from build123d import *

# Parameters (mm, degrees)
SALIENTE_EXTRUIR1_DEPTH = 111
SALIENTE_EXTRUIR2_DEPTH = 5
CROQUIS3_W              = 20
CROQUIS3_H              = 5
SALIENTE_EXTRUIR3_DEPTH = 2
SALIENTE_EXTRUIR4_DEPTH = 5
SALIENTE_EXTRUIR5_DEPTH = 2
CROQUIS6_R              = 2
CORTAR_EXTRUIR1_DEPTH   = 41
CROQUIS7_R              = 4
CORTAR_EXTRUIR2_DEPTH   = 4
CORTAR_EXTRUIR4_DEPTH   = 118


with BuildPart() as part:
    # Croquis1 → Saliente-Extruir1 (new body)
    with BuildSketch(Plane.XY):
        with BuildLine():
            Line((0, 5), (0, 0))
            Line((0, 0), (28, 0))
            ThreePointArc((28, 0), (29.414213562, 0.585786438), (30, 2))
            Line((30, 2), (30, 13))
            ThreePointArc((30, 13), (29.414213562, 14.414213562), (28, 15))
            Line((28, 15), (0, 15))
            Line((0, 15), (0, 10))
            Line((0, 10), (20, 10))
            Line((20, 10), (20, 5))
            Line((20, 5), (0, 5))
        make_face()
    extrude(amount=SALIENTE_EXTRUIR1_DEPTH)

    # Croquis2 → Saliente-Extruir2 (add)
    with BuildSketch(Plane.XY.offset(111)):
        with BuildLine():
            Line((20, 15), (20, 10))
            Line((20, 10), (20, 5))
            Line((20, 5), (0, 5))
            Line((0, 5), (0, 0))
            Line((0, 0), (28, 0))
            ThreePointArc((28, 0), (29.414213562, 0.585786438), (30, 2))
            Line((30, 2), (30, 13))
            ThreePointArc((30, 13), (29.414213562, 14.414213562), (28, 15))
            Line((28, 15), (20, 15))
        make_face()
    extrude(amount=SALIENTE_EXTRUIR2_DEPTH)

    # Croquis3 → Saliente-Extruir3 (add)
    with BuildSketch(Plane.XY.offset(116)):
        Polygon((20, 10), (20, 15), (11, 15), (0, 15), (0, 10), align=None)
        with BuildLine():
            Line((28, 15), (20, 15))
            Line((20, 15), (20, 10))
            Line((20, 10), (20, 5))
            Line((20, 5), (0, 5))
            Line((0, 5), (0, 0))
            Line((0, 0), (28, 0))
            ThreePointArc((28, 0), (29.414213562, 0.585786438), (30, 2))
            Line((30, 2), (30, 13))
            ThreePointArc((30, 13), (29.414213562, 14.414213562), (28, 15))
        make_face()
        with Locations((10, 7.5)):
            Rectangle(CROQUIS3_W, CROQUIS3_H)
    extrude(amount=SALIENTE_EXTRUIR3_DEPTH)

    # Croquis4 → Saliente-Extruir4 (add)
    with BuildSketch(Plane(origin=(0, 0, 0), x_dir=(-1, 0, 0), z_dir=(0, 0, -1))):
        with BuildLine():
            Line((-20, 5), (-20, 10))
            Line((-20, 10), (-20, 15))
            Line((-20, 15), (-28, 15))
            ThreePointArc((-28, 15), (-29.414213562, 14.414213562), (-30, 13))
            Line((-30, 13), (-30, 2))
            ThreePointArc((-30, 2), (-29.414213562, 0.585786438), (-28, 0))
            Line((-28, 0), (0, 0))
            Line((0, 0), (0, 5))
            Line((0, 5), (-20, 5))
        make_face()
    extrude(amount=SALIENTE_EXTRUIR4_DEPTH)

    # Croquis5 → Saliente-Extruir5 (add)
    with BuildSketch(Plane(origin=(0, 0, -5), x_dir=(-1, 0, 0), z_dir=(0, 0, -1))):
        with BuildLine():
            Line((0, 15), (-28, 15))
            ThreePointArc((-28, 15), (-29.414213562, 14.414213562), (-30, 13))
            Line((-30, 13), (-30, 2))
            ThreePointArc((-30, 2), (-29.414213562, 0.585786438), (-28, 0))
            Line((-28, 0), (0, 0))
            Line((0, 0), (0, 15))
        make_face()
    extrude(amount=SALIENTE_EXTRUIR5_DEPTH)

    # Croquis6 → Cortar-Extruir1 (cut)
    with BuildSketch(Plane.XZ):
        with Locations((5, 24.25)):
            Circle(CROQUIS6_R)
        with Locations((5, 86.75)):
            Circle(CROQUIS6_R)
    extrude(amount=-CORTAR_EXTRUIR1_DEPTH, mode=Mode.SUBTRACT)

    # Croquis7 → Cortar-Extruir2 (cut)
    with BuildSketch(Plane(origin=(0, 0, 0), x_dir=(-1, 0, 0), z_dir=(0, -1, 0))):
        with Locations((-5, -24.25)):
            Circle(CROQUIS7_R)
        with Locations((-5, -86.75)):
            Circle(CROQUIS7_R)
    extrude(amount=-CORTAR_EXTRUIR2_DEPTH, mode=Mode.SUBTRACT)

    # Croquis9 → Cortar-Extruir4 (cut)
    with BuildSketch(Plane.XY.offset(118)):
        Polygon((27.046454018, 15), (28.719274454, 12.085683765), (24.239354869, 9.549004814), (21.152820727, 15), align=None)
    extrude(amount=-CORTAR_EXTRUIR4_DEPTH, mode=Mode.SUBTRACT)


solid = part.part
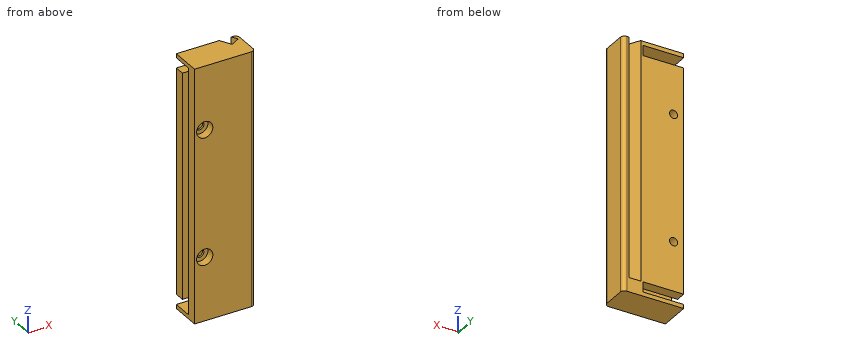
Build history of the part. All positions in model axes, mm. Give positions to 0.01 mm unless a question says otherwise; leave off trailing zeros. Loops run counter-clockwise (first coordinate to the right, second up) from the corner with the lowest first, then second, coordinate; pieces in that order, holes last. Notation, with made-up numbers: (-24.5, -32) -> (-14.5, -32) arc R18 ccw to (-14.5, -15) -> close; hole circle Ø4 at (-7, 83.5). An arc over 180 degrees is marked (long way). Answer in a Markdown table with one row per item.
Item 1: Slice it at B-B on z = 86.75. Write the cut outline in (x, y), plus the area to 3 significant figures.
Findings below:
| item | result |
|---|---|
| outline | (0, 0) -> (1, 0) -> (1, 4) -> (3, 4) -> (3, 5) -> (0, 5) -> close; (0, 10) -> (3, 10) -> (3, 15) -> (0, 15) -> close; (7, 4) -> (9, 4) -> (9, 0) -> (28, 0) arc R2 ccw to (30, 2) -> (30, 13) arc R2 ccw to (28, 15) -> (27.05, 15) -> (28.72, 12.09) -> (24.24, 9.55) -> (21.15, 15) -> (7, 15) -> (7, 10) -> (20, 10) -> (20, 5) -> (7, 5) -> close |
| area | 268 mm² |
Item 2: Slice it at A-A on x = 15. Write the cut outline in (y, z).
Findings below:
| item | result |
|---|---|
| outline | (0, -7) -> (15, -7) -> (15, -5) -> (5, -5) -> (5, 116) -> (15, 116) -> (15, 118) -> (0, 118) -> close; (10, 0) -> (15, 0) -> (15, 111) -> (10, 111) -> close |
Item 3: Slice it at C-C on y = 7.25. Write the cut outline in (x, z).
Findings below:
| item | result |
|---|---|
| outline | (0, -7) -> (30, -7) -> (30, 118) -> (0, 118) -> (0, 116) -> (20, 116) -> (20, -5) -> (0, -5) -> close |
Item 4: Probe line 1 along Z through (x, y) = (5, 12.55); line 2 along Z through (x, y) = (5, 2.3); line 3 along X through (y, z) = (2.6, 86.75). List the from-to ranges inside material, lowest first. Write a range as [from, to].
Findings below:
| item | result |
|---|---|
| line 1 | z = [-7, -5], [0, 22.25], [26.25, 84.75], [88.75, 111], [116, 118] |
| line 2 | z = [-7, 20.25], [28.25, 82.75], [90.75, 118] |
| line 3 | x = [0, 1], [9, 30] |
Item 5: Flat gauge pins, fed straight in: P1, Ø1.5, axis at y = 9, z = 67.5, coming from the -X side; P2, Ø3.5, axis at x = 5, z = 24.25, coming from the -Y side; P3, Ø2.5, axis at x = 25, y = 12.5, coming from the +Z side. Where does each tip first touch, or does it go through?
Findings below:
| item | result |
|---|---|
| P1 | stops at x = 20 |
| P2 | passes through |
| P3 | stops at z = 0 |
Item 6: Slice it at D-D on z = 60. Write the cut outline in (x, y), plus the area to 3 significant figures.
Findings below:
| item | result |
|---|---|
| outline | (0, 0) -> (28, 0) arc R2 ccw to (30, 2) -> (30, 13) arc R2 ccw to (28, 15) -> (27.05, 15) -> (28.72, 12.09) -> (24.24, 9.55) -> (21.15, 15) -> (0, 15) -> (0, 10) -> (20, 10) -> (20, 5) -> (0, 5) -> close |
| area | 324 mm² |
